```python
from build123d import *

# Parameters (mm, degrees)
SKETCH1_W           = 25.4
SKETCH1_H           = 63.5
SKETCH1_R           = 3.25755
SKETCH1_W_2         = 38.1
SKETCH1_H_2         = 25.4
BOSS_EXTRUDE1_DEPTH = 6
FILLET1_R           = 10


with BuildPart() as part:
    # Sketch1 → Boss-Extrude1 (new body)
    with BuildSketch(Plane(origin=(0, 0, 0), x_dir=(1, 0, 0), z_dir=(0, 1, 0))):
        with Locations((12.7, 31.75)):
            Rectangle(SKETCH1_W, SKETCH1_H)
        with Locations((12.7, 12.7)):
            Circle(SKETCH1_R, mode=Mode.SUBTRACT)
        with Locations((12.7, 51.5)):
            Circle(SKETCH1_R, mode=Mode.SUBTRACT)
        with Locations((44.45, 12.7)):
            Rectangle(SKETCH1_W_2, SKETCH1_H_2)
        with Locations((50.8, 12.7)):
            Circle(SKETCH1_R, mode=Mode.SUBTRACT)
    extrude(amount=BOSS_EXTRUDE1_DEPTH)

    # Fillet1
    fillet1_edges = [part.edges().sort_by_distance(p)[0] for p in [
        (0, 3, 0),
        (0, 3, -63.5),
        (25.4, 3, -63.5),
        (25.4, 3, -25.4),
        (63.5, 3, -25.4),
        (63.5, 3, 0),
    ]]
    fillet(fillet1_edges, radius=FILLET1_R)


solid = part.part
```
Geometry: final body of the model. Coordinates: model frame, mm. A direction names the side the tool comes from. Coordinates: 2 decimals unless noted, no trailing zeros. Order: outer loops, then holes, each group sorted by start corner. A loop starts at its lowest first (then second) coordinate and runs counter-clockwise, first axis right, second up. Notation, with made-up numbers: M 27,33.5 L 57,33.5 A36 cw 57,68.5 Z; hole C -38,-8 d9. An arc over 180 degrees is marked long. Answer as CSV lines item,"result".
Q1. Section C-C on z = -12.7. Return the cut outline in (x, y).
Answers:
outline,"M 0,0 L 9.44,0 L 9.44,6 L 0,6 Z; M 15.96,0 L 47.54,0 L 47.54,6 L 15.96,6 Z; M 54.06,0 L 63.5,0 L 63.5,6 L 54.06,6 Z"
Q2. Section A-A on z = -51.5. Return the cut outline in (x, y).
Answers:
outline,"M 0,0 L 9.44,0 L 9.44,6 L 0,6 Z; M 15.96,0 L 25.4,0 L 25.4,6 L 15.96,6 Z"
Q3. Section D-D on x = 12.7. Return the cut outline in (y, z).
Answers:
outline,"M 0,-63.5 L 6,-63.5 L 6,-54.76 L 0,-54.76 Z; M 0,-48.24 L 6,-48.24 L 6,-15.96 L 0,-15.96 Z; M 0,-9.44 L 6,-9.44 L 6,0 L 0,0 Z"
Q4. Set-up query: faces 4 (the cylindrical face through (47.546, 2.958, -12.843)), 5 (the flat face through (25.4, 3, -44)). Return all of +Z, -Z, +X, -X, +Y, -Y with unobstructed straight access to the full face (end or side cutting, diameter ignored); none if empty.
Answers:
face 4,"+Y, -Y"
face 5,"-Z, +X, +Y, -Y"
Q5. Section B-B on x = 50.8. Return the cut outline in (y, z), and give its area (3 significant figures).
Answers:
outline,"M 0,-25.4 L 6,-25.4 L 6,-15.96 L 0,-15.96 Z; M 0,-9.44 L 6,-9.44 L 6,0 L 0,0 Z"
area,"113 mm^2"
Q6. First-contact query: P1, Ø1.5, axis at y = 1, z = -22, coming from the +X side; P2, Ø3, axis at y = 4.5, z = -48, coming from the +X side; P3, Ø6, axis at x = 12.7, z = -12.7, coming from the -Y side. Flat tips, straight axial feed; report the tip coordinate or a pass-through.
Answers:
P1,"stops at x = 61.61"
P2,"stops at x = 25.4"
P3,"passes through"
Q7. Draft query along X for faces 1 (the flat face through (63.5, 3, -13)), 2 (the flat face through (0, 3, -31)), 3 (the cylindrical face through (9.446, 2.958, -51.643)). Return one class per face: pulls with the +X half, pulls with the -X half, needs draft (parallel to the pull), parting line crosses it, or undercut.
Answers:
face 1,"pulls with the +X half"
face 2,"pulls with the -X half"
face 3,"undercut"
Q8. Line query: probe 1 along X at (y, z) = (2.2, -12.7); probe 2 along Z at (x, y) = (12.7, 1.8); probe 3 along Z at (x, y) = (50.8, 1.95). Output: solid intervals per line, ascending. Write a range as [from, to].
Answers:
probe 1,"x = [0, 9.44], [15.96, 47.54], [54.06, 63.5]"
probe 2,"z = [-63.5, -54.76], [-48.24, -15.96], [-9.44, 0]"
probe 3,"z = [-25.4, -15.96], [-9.44, 0]"
